Read the model definition and answer for the solid it produces. Units are mm, in the model's axes. A direction names the side the tool comes from. Give positions to 0.01 mm unless a question says otherwise; leave off trailing zeros. Write each loop counter-clockwise with the first axis right and the second up, starting at its lowest first coordinate (ties: lowest second). Pieces come first, ordered by that corner, then holes. Notation, with made-up numbers: (19, 71) -> (25, 71) arc R26 ccw to (25, 110) -> close; hole circle Ø5 at (-7.5, -37). An arc over 180 degrees is marked (long way). Write item = value, one per line.
Autodesk Inventor part; units mm, degrees
ref_plane "YZ Plane" through (0, 0, 0) normal (1, 0, 0) x (0, 1, 0)
ref_plane "XZ Plane" through (0, 0, 0) normal (0, 1, 0) x (-1, 0, 0)
ref_plane "XY Plane" through (0, 0, 0) normal (0, 0, 1) x (1, 0, 0)
sketch "Sketch1" plane through (0, 0, 0) normal (0, 1, 0) x (-1, 0, 0)
  line L0 (0, 25.4) -> (25.4, 25.4)
  line L1 (25.4, 25.4) -> (25.4, 0)
  line L2 (25.4, 0) -> (0, 0)
  line L3 (0, 0) -> (0, 25.4)
  line L4 (22.225, 22.225) -> (3.175, 22.225)
  line L5 (3.175, 22.225) -> (3.175, 3.175)
  line L6 (3.175, 3.175) -> (22.225, 3.175)
  line L7 (22.225, 3.175) -> (22.225, 22.225)
  dimension "d0" = 25.4
  dimension "d1" = 25.4
  dimension "d2" = 3.175
extrude "Extrusion1" add sketch "Sketch1" along normal blind 558.8
sketch "Sketch2" plane through (-25.4, 0, 25.4) normal (0, 0, 1) x (1, 0, 0)
  line L0 (25.4, 0) -> (0, 0)
  line L1 (0, 558.8) -> (25.4, 558.8)
  line L2 (12.7, 558.8) -> (12.7, 0) construction
  line L3 (12.7, 0) -> (12.7, 13.97) construction
  circle A0 centre (12.7, 13.97) radius 3.302
  circle A1 centre (12.7, 33.6315) radius 3.302
  circle A2 centre (12.7, 53.293) radius 3.302
  circle A3 centre (12.7, 72.9544) radius 3.302
  circle A4 centre (12.7, 92.6159) radius 3.302
  circle A5 centre (12.7, 112.2774) radius 3.302
  circle A6 centre (12.7, 131.9389) radius 3.302
  circle A7 centre (12.7, 151.6004) radius 3.302
  circle A8 centre (12.7, 171.2619) radius 3.302
  circle A9 centre (12.7, 190.9233) radius 3.302
  circle A10 centre (12.7, 210.5848) radius 3.302
  circle A11 centre (12.7, 230.2463) radius 3.302
  circle A12 centre (12.7, 249.9078) radius 3.302
  circle A13 centre (12.7, 269.5693) radius 3.302
  circle A14 centre (12.7, 289.2307) radius 3.302
  circle A15 centre (12.7, 308.8922) radius 3.302
  circle A16 centre (12.7, 328.5537) radius 3.302
  circle A17 centre (12.7, 348.2152) radius 3.302
  circle A18 centre (12.7, 367.8767) radius 3.302
  circle A19 centre (12.7, 387.5381) radius 3.302
  circle A20 centre (12.7, 407.1996) radius 3.302
  circle A21 centre (12.7, 426.8611) radius 3.302
  circle A22 centre (12.7, 446.5226) radius 3.302
  circle A23 centre (12.7, 466.1841) radius 3.302
  circle A24 centre (12.7, 485.8456) radius 3.302
  circle A25 centre (12.7, 505.507) radius 3.302
  circle A26 centre (12.7, 525.1685) radius 3.302
  circle A27 centre (12.7, 544.83) radius 3.302
  dimension "d5" = 13.97
  dimension "d6" = 6.604
  dimension "d7" = 558.8
  dimension "d10" = 19.6615
extrude "Extrusion2" [suppressed]
sketch "Sketch3" plane through (-25.4, 0, 0) normal (-1, 0, 0) x (0, 0, 1)
  line L0 (25.4, 0) -> (25.4, 558.8)
  line L1 (0, 0) -> (0, 558.8)
  line L2 (0, 210.5848) -> (25.4, 210.5848) construction
  line L3 (12.7, 498.5456) -> (12.7, 454.0956) construction
  line L4 (12.7, 373.6152) -> (12.7, 322.8152) construction
  line L5 (12.7, 232.8098) -> (12.7, 188.3598) construction
  line L6 (12.7, 104.7044) -> (12.7, 60.2544) construction
  circle A0 centre (12.7, 498.5456) radius 3.302
  circle A1 centre (12.7, 454.0956) radius 3.302
  circle A2 centre (12.7, 373.6152) radius 3.302
  circle A3 centre (12.7, 322.8152) radius 3.302
  circle A4 centre (12.7, 232.8098) radius 3.302
  circle A5 centre (12.7, 188.3598) radius 3.302 construction
  circle A6 centre (12.7, 104.7044) radius 3.302
  circle A7 centre (12.7, 60.2544) radius 3.302
  line L7 (0, 279.4) -> (25.4, 279.4) construction
  line L8 (12.7, 304.8) -> (12.7, 254) construction
  circle A8 centre (12.7, 304.8) radius 3.302
  circle A9 centre (12.7, 254) radius 3.302
  line L9 (25.4, 0) -> (0, 0)
  line L10 (0, 558.8) -> (25.4, 558.8)
  circle A10 centre (12.7, 546.1) radius 3.302
  line L11 (12.7, 546.1) -> (12.7, 558.8) construction
  line L12 (12.7, 0) -> (12.7, 12.7) construction
  circle A11 centre (12.7, 12.7) radius 3.302
  line L13 (0, 82.4794) -> (25.4, 82.4794) construction
  line L14 (0, 476.3206) -> (25.4, 476.3206) construction
  line L15 (12.7, 12.7) -> (12.7, 34.8544) construction
  circle A12 centre (12.7, 34.8544) radius 3.302
  line L16 (0, 13.97) -> (25.4, 13.97) construction
  line L17 (0, 33.6315) -> (25.4, 33.6315) construction
  line L18 (0, 53.293) -> (25.4, 53.293) construction
  line L19 (0, 72.9544) -> (25.4, 72.9544) construction
  line L20 (0, 92.6159) -> (25.4, 92.6159) construction
  line L21 (0, 112.2774) -> (25.4, 112.2774) construction
  line L22 (0, 131.9389) -> (25.4, 131.9389) construction
  line L23 (0, 151.6004) -> (25.4, 151.6004) construction
  line L24 (0, 171.2619) -> (25.4, 171.2619) construction
  line L25 (0, 190.9233) -> (25.4, 190.9233) construction
  line L26 (0, 210.5848) -> (25.4, 210.5848) construction
  line L27 (0, 230.2463) -> (25.4, 230.2463) construction
  line L28 (0, 249.9078) -> (25.4, 249.9078) construction
  line L29 (0, 269.5693) -> (25.4, 269.5693) construction
  line L30 (0, 289.2307) -> (25.4, 289.2307) construction
  line L31 (0, 308.8922) -> (25.4, 308.8922) construction
  line L32 (0, 328.5537) -> (25.4, 328.5537) construction
  line L33 (0, 348.2152) -> (25.4, 348.2152) construction
  line L34 (0, 367.8767) -> (25.4, 367.8767) construction
  line L35 (0, 387.5381) -> (25.4, 387.5381) construction
  line L36 (0, 407.1996) -> (25.4, 407.1996) construction
  line L37 (0, 426.8611) -> (25.4, 426.8611) construction
  line L38 (0, 446.5226) -> (25.4, 446.5226) construction
  line L39 (0, 466.1841) -> (25.4, 466.1841) construction
  line L40 (0, 485.8456) -> (25.4, 485.8456) construction
  line L41 (0, 505.507) -> (25.4, 505.507) construction
  line L42 (0, 525.1685) -> (25.4, 525.1685) construction
  line L43 (0, 544.83) -> (25.4, 544.83) construction
  point P0 (12.7, 279.4)
  point P1 (12.7, 82.4794)
  point P2 (12.7, 476.3206)
  point P3 (12.7, 348.2152)
  point P4 (12.7, 210.5848)
  dimension "d17" = 44.45
  dimension "d18" = 50.8
  dimension "d19" = 44.45
  dimension "d20" = 44.45
  dimension "d21" = 6.604
  dimension "d22" = 6.604
  dimension "d23" = 6.604
  dimension "d24" = 6.604
  dimension "d25" = 6.604
  dimension "d26" = 6.604
  dimension "d27" = 6.604
  dimension "d28" = 6.604
  dimension "d31" = 50.8
  dimension "d32" = 6.604
  dimension "d33" = 6.604
  dimension "d40" = 12.7
  dimension "d41" = 6.604
  dimension "d42" = 12.7
  dimension "d43" = 6.604
  dimension "d64" = 25.4
  dimension "d65" = 6.604
  dimension "d66" = 13.97
  dimension "d67" = 558.8
  dimension "d70" = 19.6615
  dimension "d76" = 9.525
  dimension "d77" = 9.525
extrude "Extrusion3" cut sketch "Sketch3" against normal through all contours A0 | A1 | A6 | A7 | A8 | A9 | A10 | A11 | A12
sketch "Sketch4" plane through (0, 0, 25.4) normal (1, 0, 0) x (0, 0, -1)
  circle A0 centre (12.7, 304.8) radius 3.302 construction
  circle A1 centre (12.7, 254) radius 3.302 construction
  line L0 (0, 0) -> (0, 558.8)
  line L1 (12.7, 304.8) -> (12.7, 323.85) construction
  line L2 (12.7, 254) -> (12.7, 234.95) construction
  circle A2 centre (12.7, 323.85) radius 3.302
  circle A3 centre (12.7, 234.95) radius 3.302
  line L3 (25.4, 0) -> (0, 0)
  line L4 (0, 558.8) -> (25.4, 558.8)
  line L5 (12.7, 558.8) -> (12.7, 0) construction
  circle A4 centre (12.7, 419.1) radius 3.302
  circle A5 centre (12.7, 400.05) radius 3.302
  circle A6 centre (12.7, 381) radius 3.302
  circle A7 centre (12.7, 361.95) radius 3.302
  circle A8 centre (12.7, 342.9) radius 3.302
  circle A9 centre (12.7, 431.8) radius 3.302
  circle A10 centre (12.7, 215.9) radius 3.302
  circle A11 centre (12.7, 196.85) radius 3.302
  circle A12 centre (12.7, 177.8) radius 3.302
  circle A13 centre (12.7, 158.75) radius 3.302
  circle A14 centre (12.7, 139.7) radius 3.302
  dimension "d46" = 19.05
  dimension "d47" = 19.05
  dimension "d48" = 6.604
  dimension "d49" = 6.604
  dimension "d52" = 6.604
  dimension "d53" = 139.7
  dimension "d80" = 19.05
  dimension "d85" = 12.7
  dimension "d88" = 19.05
extrude "Extrusion4" cut sketch "Sketch4" against normal blind 25.4
equation "\"d19\" = d17"
equation "\"d20\" = d17"
equation "\"d22\" = d21"
equation "\"d23\" = d21"
equation "\"d24\" = d21"
equation "\"d25\" = d21"
equation "\"d26\" = d21"
equation "\"d27\" = d21"
equation "\"d28\" = d21"
equation "\"d31\" = d18"
equation "\"d32\" = d21"
equation "\"d33\" = d21"
equation "\"d41\" = d21"
equation "\"d42\" = d40"
equation "\"d43\" = d21"
equation "\"d70\" = -0.0740741 * d66 + 0.037037 * d67"
equation "\"d76\" = d77"
properties part number "Chassis V1.500 Part4" material "Aluminum 6061"
(1) For a pull along Z with two mould halves and no side action, classify faces 1 (the flat face through (-24, 0, 13)), 2 (the flat face through (-13, 275, 25.4)), 3 (the flat face through (-13, 275, 22.225)), 4 (the flat face through (-22.225, 275, 13)) as released by +Z, released by -Z, zero draft, split by the parting line, or undercut.
Checks:
face_1 = zero draft
face_2 = released by +Z
face_3 = undercut
face_4 = undercut
(2) The part is cut by section A-A on x = -8.5. Determine the outline of the cut face in (y, z) (3 decimals), plus the area to 3 significant figures.
Checks:
outline = (0, 0) -> (558.8, 0) -> (558.8, 3.175) -> (0, 3.175) -> close; (0, 22.225) -> (558.8, 22.225) -> (558.8, 25.4) -> (0, 25.4) -> close
area = 3,550 mm²
(3) A tool of negligible diameter and unlimited length cuts with its end or side. For faces 5 (the flat face through (-24, 558.8, 13)), 6 (the flat face through (-13, 275, 3.175)), from which of +Z, -Z, +X, -X, +Y, -Y can it reach the whole face along a straight path? Write none if from no direction.
Checks:
face_5 = +Z, -Z, +X, -X, +Y
face_6 = +Y, -Y
(4) Given P1, Ø7.5, axis at y = 177.8, z = 12.7, coming from the -X side; P2, Ø4, axis at y = 454.1, z = 12.7, coming from the +X side, each flat-ended and moving along its own axis, determine where each tip first touches the part or whether it passes through.
Checks:
P1 = -25.4
P2 = through
(5) Consider L1, parallel to X at y = 71.5, z = 19.25 (3 decimals); L2, parallel to Z at x = -21.5, y = 443.5 (3 decimals); L3, parallel to Z at x = -24.4, y = 234.95. Determine where each line is inside the solid, lowest interval first.
Checks:
L1 = -25.4 to -22.225, -3.175 to 0
L2 = 0 to 3.175, 22.225 to 25.4
L3 = 0 to 9.4, 16 to 25.4
(6) The part is cut by section B-B on y = 93. Determine the outline of the cut face in (x, z) (3 decimals).
Checks:
outline = (-25.4, 0) -> (0, 0) -> (0, 25.4) -> (-25.4, 25.4) -> close; hole (-22.225, 3.175) -> (-3.175, 3.175) -> (-3.175, 22.225) -> (-22.225, 22.225) -> close
